Verification items for the finished model (mm, model axes). A direction names the side the tool comes from. Coordinates: 2 decimals unless noted, no trailing zeros. Order: outer loops, then holes, each group sorted by start corner. A loop starts at its lowest first (then second) coordinate and runs counter-clockwise, first axis right, second up. Notation, with made-up numbers: (12, 59) -> (49, 59) arc R22 cw to (49, 68) -> close; hole circle Ø5 at (53.5, 11). An arc over 180 degrees is marked (long way). Write each question's results on one line, items separated by ' | '. Start each with the question number.
(1) Cross-section at C-C on x = 2.2. Give the number of separate pieces and of enclosed holes in the cut face, and give its area (3 significant figures).
(2) Thickness scan on probe 1 along Y at (x, z) = (1.8, -4); probe 2 along X at (y, z) = (5.5, 7); probe 3 along Z at (x, y) = (2.15, 3.5). Record the ranges inside material, lowest first. Write a range as [from, to].
(3) Set-up check for faces 1 (the cylindrical face through (1.52, 0.07, 1.5)), 2 (the flat face through (3, 4, 4)), 3 (the cylindrical face through (2.014, -3.537, -9.168)): record each of +Z, -Z, +X, -X, +Y, -Y from which the full face is reachable in a straight line by a thin tool's end or side.
(4) Cross-section at A-A on z = 0. Enter the section's corners in (x, y), and give its area (3 significant figures).
(5) Draft check along Z on faces 4 (the cylindrical face through (2, 10, 0)), 5 (the cylindrical face through (2, -0.6, -10.2)), 6 (the flat face through (5, 1.2, 0.1)), 7 (the cylindrical face through (1.986, -14.985, 0.66)). Enter one of: +Z half, -Z half, draft (parallel to the pull), parting line (faces both ways), or undercut.
(6) Cross-section at D-D on x = 4.4. Enter the section's corners in (y, z), and give its area (3 significant figures).
(7) Go/stop test with flat-tipped pins: pin 1 (2.5 mm diameter, centred on y = 0, z = -11, fed in from -X); pin 2 (3 mm diameter, centred on x = 1.5, y = -6.5, fed in from +Z); pin 3 (2.5 mm diameter, centred on y = 0, z = 11, fed in from +X). Record where each tip stops, or that it passes through.
```python
from build123d import *

# Parameters (mm, degrees)
SKETCH3_R           = 1.5
EXTRUDE1_DEPTH      = 4
SKETCH4_R           = 1
SKETCH4_R_2         = 1.25
EXTRUDE2_DEPTH      = 4
SKETCH5_R           = 5
SKETCH5_R_2         = 1
BOSS_EXTRUDE1_DEPTH = 2
SKETCH6_R           = 15
SKETCH6_R_2         = 5
CUT_EXTRUDE2_DEPTH  = 1


with BuildPart() as part:
    # Sketch1 → Revolve1 (revolve)
    with BuildSketch(Plane.XY):
        Polygon((1.809375, 15), (1.190625, 15), (0, 15), (0, 14), (0, 0), (3, 0), (3, 14), (3, 15), align=None)
    revolve(axis=Axis((0, 0, 0), (1, 0, 0)))

    # Sketch3 → Extrude1 (cut, through all)
    with BuildSketch(Plane(origin=(3, 0, 0), x_dir=(0, 0, -1), z_dir=(1, 0, 0))):
        Circle(SKETCH3_R)
    extrude(amount=-EXTRUDE1_DEPTH, mode=Mode.SUBTRACT)

    # Sketch4 → Extrude2 (cut, through all)
    with BuildSketch(Plane(origin=(3, 0, 0), x_dir=(0, 0, -1), z_dir=(1, 0, 0))):
        with Locations((0, 11)):
            Circle(SKETCH4_R)
        with Locations((-4.381841494, 10.089572098)):
            Circle(SKETCH4_R_2)
        with Locations((4.381841494, 10.089572098)):
            Circle(SKETCH4_R_2)
        with Locations((10.089572098, -4.381841494)):
            Circle(SKETCH4_R_2)
        with Locations((11, 0)):
            Circle(SKETCH4_R)
        with Locations((10.089572098, 4.381841494)):
            Circle(SKETCH4_R_2)
        with Locations((-4.381841494, -10.089572098)):
            Circle(SKETCH4_R_2)
        with Locations((0, -11)):
            Circle(SKETCH4_R)
        with Locations((4.381841494, -10.089572098)):
            Circle(SKETCH4_R_2)
        with Locations((-10.089572098, 4.381841494)):
            Circle(SKETCH4_R_2)
        with Locations((-11, 0)):
            Circle(SKETCH4_R)
        with Locations((-10.089572098, -4.381841494)):
            Circle(SKETCH4_R_2)
    extrude(amount=-EXTRUDE2_DEPTH, mode=Mode.SUBTRACT)

    # Sketch5 → Boss-Extrude1 (add)
    with BuildSketch(Plane(origin=(3, 0, 0), x_dir=(0, 0, -1), z_dir=(1, 0, 0))):
        Circle(SKETCH5_R)
        Circle(SKETCH5_R_2, mode=Mode.SUBTRACT)
    extrude(amount=BOSS_EXTRUDE1_DEPTH)

    # Sketch6 → Cut-Extrude2 (cut)
    with BuildSketch(Plane.ZY):
        Circle(SKETCH6_R)
        Circle(SKETCH6_R_2, mode=Mode.SUBTRACT)
    extrude(amount=-CUT_EXTRUDE2_DEPTH, mode=Mode.SUBTRACT)


solid = part.part
```
Results are:
1) separate pieces: 1 | enclosed holes: 13 | area: 648 mm2
2) probe 1: y = [-14.46, -11.28], [-8.9, 8.9], [11.28, 14.46] | probe 2: x = [1, 3] | probe 3: z = [-14.59, -10.98], [-9.2, 9.2], [10.98, 14.59]
3) face 1: -X | face 2: +X | face 3: +X, -X
4) outline: (0, -5) -> (1, -5) -> (1, -10) -> (3, -10) -> (3, -5) -> (5, -5) -> (5, -1) -> (3, -1) -> (3, -1.5) -> (0, -1.5) -> close; (0, 1.5) -> (3, 1.5) -> (3, 1) -> (5, 1) -> (5, 5) -> (3, 5) -> (3, 10) -> (1, 10) -> (1, 5) -> (0, 5) -> close; (1, -15) -> (3, -15) -> (3, -12) -> (1, -12) -> close; (1, 12) -> (3, 12) -> (3, 15) -> (1, 15) -> close | area: 69.0 mm2
5) face 4: undercut | face 5: undercut | face 6: draft | face 7: parting line
6) outline: circle Ø10 at (0, 0); hole circle Ø2 at (0, 0) | area: 75.4 mm2
7) pin 1: stops at x = 1 | pin 2: stops at z = 14.14 | pin 3: stops at x = 3
